from build123d import *

# Parameters (mm, degrees)
BOSS_EXTRUDE1_DEPTH = 2
SKETCH2_R           = 5
BOSS_EXTRUDE2_DEPTH = 15
SKETCH4_R           = 4
CUT_EXTRUDE1_DEPTH  = 10
SKETCH5_R           = 2.5
BOSS_EXTRUDE3_DEPTH = 22


with BuildPart() as part:
    # Sketch1 → Boss-Extrude1 (new body)
    with BuildSketch(Plane.XY):
        with BuildLine():
            Line((-22.5, -7.5), (22.5, -7.5))
            ThreePointArc((22.5, -7.5), (23.959503782, 0), (22.5, 7.5))
            Line((22.5, 7.5), (-22.5, 7.5))
            ThreePointArc((-22.5, 7.5), (-23.959503782, 0), (-22.5, -7.5))
        make_face()
    extrude(amount=BOSS_EXTRUDE1_DEPTH)

    # Sketch2 → Boss-Extrude2 (add)
    with BuildSketch(Plane.XY.offset(2)):
        Circle(SKETCH2_R)
    extrude(amount=BOSS_EXTRUDE2_DEPTH)

    # Sketch4 → Cut-Extrude1 (cut)
    with BuildSketch(Plane.XY.offset(17)):
        Circle(SKETCH4_R)
    extrude(amount=-CUT_EXTRUDE1_DEPTH, mode=Mode.SUBTRACT)

    # Sketch5 → Boss-Extrude3 (add)
    with BuildSketch(Plane.XY.offset(2)):
        with Locations((-17, 0)):
            Circle(SKETCH5_R)
        with Locations((17, 0)):
            Circle(SKETCH5_R)
    extrude(amount=BOSS_EXTRUDE3_DEPTH)


solid = part.part
Can you work these out from the model? Positions are in its coordinate system, mm. A direction names the side the tool comes from. Coordinates: 2 decimals unless noted, no trailing zeros. Write each loop counter-clockwise with the first axis right and the second up, starting at its lowest first coordinate (ties: lowest second). Pieces come first, ordered by that corner, then holes. Notation, with made-up numbers: (-39.75, 33.25) - (-24.75, 33.25) arc R11 cw to (-24.75, 49.25) - close; hole circle Ø7 at (17.25, 57). An arc over 180 degrees is marked (long way). Return JSON: item names as keys, results as strings. Group by question number.
Item 1: If we section it at C-C (z = 12.25): Write out the boundary of the cut face in (x, y), then the cut area to 3 significant figures.
Item 2: I'm going to push flat-ended pins straight in: pin 1 Ø4 at (x, z) = (3.5, 5) entering from +Y; pin 2 Ø8 at (y, z) = (3.5, 18.5) entering from -X; pin 3 Ø12 at (x, z) = (13.5, 6.5) entering from +Y; pin 4 Ø8 at (x, y) = (-1.5, -0.5) entering from +Z. Where does each tip first touch, or does it pass through?
Item 3: We'd pull the mould along X, two halves only. Please class faces 1 (the face through (14.5, 0.1, 12.8)), 2 (the face through (23.96, -0.11, 0.99)), 3 (the face through (0, 7.5, 1)), 4 (the face through (-23.96, 0.11, 0.99)): pulls with the +X half, pulls with the -X half, needs draft (parallel to the pull), parting line crosses it, or undercut.
Item 4: If we section it at B-B (y = 0): Write out the boundary of the cut face in (x, z).
Item 5: If we section it at A-A (x = 17): Write out the boundary of the cut face in (y, z).
Item 6: Which directions (+Z, -Z, +X, -X, +Y, -Y) give clear straight access to the entire face, cutting with the end or side of a thin tool? Please do faces 5 (the face through (17, 0, 24)), 6 (the face through (-0.867, -3.905, 12.07)).
Item 7: Please list where these lines run through material, in increasing order: probe 1 along Y at (x, z) = (0, 14); probe 2 along X at (y, z) = (-0.5, 13.5); probe 3 along X at (y, z) = (2, 15.25).
Item 8: If we section it at D-D (z = 18): Write out the boundary of the cut face in (x, y).
Return value:
{
 "1": {"outline": "circle Ø5 at (-17, 0); circle Ø10 at (0, 0); circle Ø5 at (17, 0); hole circle Ø8 at (0, 0)", "area": "67.5 mm^2"},
 "2": {"pin 1": "stops at y = 4.77", "pin 2": "stops at x = -19.5", "pin 3": "stops at y = 7.5", "pin 4": "stops at z = 17"},
 "3": {"face 1": "undercut", "face 2": "pulls with the +X half", "face 3": "needs draft", "face 4": "pulls with the -X half"},
 "4": {"outline": "(-23.96, 0) - (23.96, 0) - (23.96, 2) - (19.5, 2) - (19.5, 24) - (14.5, 24) - (14.5, 2) - (5, 2) - (5, 17) - (4, 17) - (4, 7) - (-4, 7) - (-4, 17) - (-5, 17) - (-5, 2) - (-14.5, 2) - (-14.5, 24) - (-19.5, 24) - (-19.5, 2) - (-23.96, 2) - close"},
 "5": {"outline": "(-7.5, 0) - (7.5, 0) - (7.5, 2) - (2.5, 2) - (2.5, 24) - (-2.5, 24) - (-2.5, 2) - (-7.5, 2) - close"},
 "6": {"face 5": "+Z, +X, -X, +Y, -Y", "face 6": "+Z"},
 "7": {"probe 1": "y = -5 to -4, 4 to 5", "probe 2": "x = -19.45 to -14.55, -4.97 to -3.97, 3.97 to 4.97, 14.55 to 19.45", "probe 3": "x = -18.5 to -15.5, -4.58 to -3.46, 3.46 to 4.58, 15.5 to 18.5"},
 "8": {"outline": "circle Ø5 at (-17, 0); circle Ø5 at (17, 0)"}
}
